```python
from build123d import *

# Parameters (mm, degrees)
PAD_DEPTH       = 4
PAD_DEPTH_BACK  = 4
SKETCH001_R     = 1.75
POCKET_DEPTH    = 6.001
CHAMFER_SIZE    = 1
POCKET001_DEPTH = 2.5
CHAMFER001_SIZE = 1


with BuildPart() as part:
    # Sketch → Pad (new body, two sides)
    with BuildSketch(Plane.XY) as pad_sk:
        with BuildLine():
            Line((-16, 0), (-20, 0))
            Line((-20, 0), (-20, 6))
            Line((-20, 6), (4, 6))
            Line((4, 6), (4, 0))
            Line((-4, 0), (4, 0))
            Line((-4, 0), (-4, 1))
            ThreePointArc((-4, 1), (-4.87868, 3.12132), (-7, 4))
            Line((-13, 4), (-7, 4))
            ThreePointArc((-13, 4), (-15.12132, 3.12132), (-16, 1))
            Line((-16, 0), (-16, 1))
        make_face()
    extrude(amount=PAD_DEPTH)
    extrude(pad_sk.sketch, amount=-PAD_DEPTH_BACK)

    # Sketch001 → Pocket (cut, through all)
    with BuildSketch(Plane.XZ):
        Circle(SKETCH001_R)
    extrude(amount=-POCKET_DEPTH, mode=Mode.SUBTRACT)

    # Chamfer
    chamfer_edges = [part.edges().sort_by_distance(p)[0] for p in [
        (-20, 3, 4),
        (4, 3, 4),
        (4, 3, -4),
        (-20, 3, -4),
    ]]
    chamfer(chamfer_edges, length=CHAMFER_SIZE)

    # Sketch002 (on DatumPlane) → Pocket001 (cut)
    with BuildSketch(Plane(origin=(0, 6, 0), x_dir=(-1, 0, 0), z_dir=(0, 1, 0))):
        Polygon((3.233162, 0), (1.616581, 2.8), (-1.616581, 2.8), (-3.233162, 0), (-1.616581, -2.8), (1.616581, -2.8), align=None)
    extrude(amount=-POCKET001_DEPTH, mode=Mode.SUBTRACT)

    # Chamfer001
    chamfer001_edges = [part.edges().sort_by_distance(p)[0] for p in [
        (-4, 0.5, 4),
        (-4, 0.5, -4),
    ]]
    chamfer(chamfer001_edges, length=CHAMFER001_SIZE)


solid = part.part
```
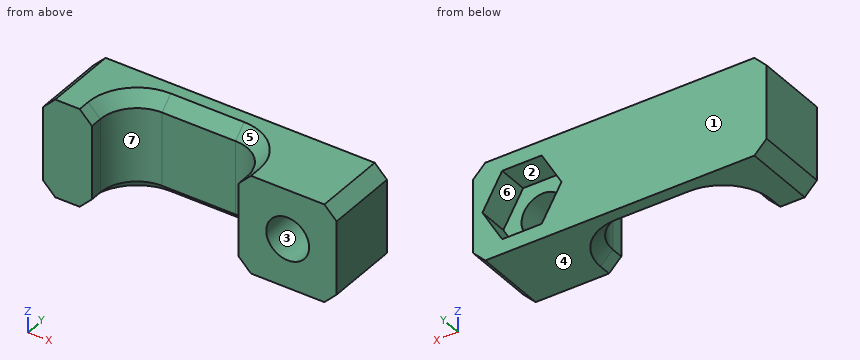
For this review, take the finished solid that the model builds, in its own axes (mm). Face numbers are marked on the shaded views. A direction names the side the tool comes from. Round coordinates to 2 decimals unless told otherwise and drop trailing zeros. Write each loop counter-clockwise with the first axis right and the second up, starting at its lowest first coordinate (ties: lowest second). Pieces come first, ordered by that corner, then holes. Notation, with made-up numbers: (72.25, 73) -> (131.25, 73) arc R17 ccw to (131.25, 81) -> close; hole circle Ø7 at (57.25, 74.25). An arc over 180 degrees is marked (long way). One line per question, with ' | ' between items. Start each with the question number.
1) For pin 1 Ø3 at (x, z) = (-11, 0) entering from -Y, flat-tipped, find the tip position at first contact; note if it passes through.
2) Mouldability with a two-part tool opening along Z and no side actions: class the marked faces 1, 2, 3 and 4 as +Z half, -Z half, draft (parallel to the pull), parting line (faces both ways), or undercut.
3) Wall thickness on line 1 along X through (y, z) = (4.35, -0.75); line 2 along Z through (x, y) = (0, 3.25); line 3 along Y through (x, z) = (-8.5, 0.75): over which ranges is each line inside the solid? List them lowest first.
4) Add section A-A (x = 0). Write out the cut boundary in (y, z), and give its area (4 significant figures).
5) Add section C-C (x = -8.5). Write out the cut boundary in (y, z), and give its area (3 significant figures).
6) Add section D-D (y = 2.75). Count the separate pieces of the cut face and the enclosed holes in it, and give its area (3 significant figures).
7) Add section B-B (z = 1.5). Write out the cut boundary in (x, y).
8) Machinability: for the marked faces 5, 6 and 7, which of the approach directions +Z, -Z, +X, -X, +Y, -Y give a long, thin tool a straight path to every point of the face, cutting with its end or side? Answer none if there is none.
Reported:
1) pin 1: stops at y = 4
2) face 1: draft | face 2: undercut | face 3: undercut | face 4: -Z half
3) line 1: x = -20 to -2.8, 2.8 to 4 | line 2: z = -4 to -1.75, 1.75 to 4 | line 3: y = 4 to 6
4) outline: (0, -4) -> (6, -4) -> (6, -2.8) -> (3.5, -2.8) -> (3.5, -1.75) -> (0, -1.75) -> close; (0, 1.75) -> (3.5, 1.75) -> (3.5, 2.8) -> (6, 2.8) -> (6, 4) -> (0, 4) -> close | area: 21.75 mm²
5) outline: (4, -3) -> (5, -4) -> (6, -4) -> (6, 4) -> (5, 4) -> (4, 3) -> close | area: 15.0 mm²
6) separate pieces: 2 | enclosed holes: 1 | area: 91.0 mm²
7) outline: (-20, 0) -> (-16, 0) -> (-16, 1) arc R3 cw to (-13, 4) -> (-7, 4) arc R3 cw to (-4, 1) -> (-4, 0) -> (-0.9, 0) -> (-0.9, 3.5) -> (-2.37, 3.5) -> (-2.37, 6) -> (-20, 6) -> close; (0.9, 0) -> (4, 0) -> (4, 6) -> (2.37, 6) -> (2.37, 3.5) -> (0.9, 3.5) -> close
8) face 5: +Z, -Y | face 6: +Y | face 7: +Z, -Z, -Y
